Here's how the part is built. I have some questions about the finished solid (model axes, mm). A direction names the side the tool comes from. Coordinates: 2 decimals unless noted, no trailing zeros. Loops run counter-clockwise (first coordinate to the right, second up) from the corner with the lowest first, then second, coordinate; pieces in that order, holes last.
from build123d import *

# Parameters (mm, degrees)
SKETCH_1_W                  = 2300
SKETCH_1_H                  = 132
SM_BASE_FLANGE_1_DEPTH      = 1.6
SM_EDGE_FLANGE_1_DEPTH      = 2200
SM_EDGE_FLANGE_1_BEND_DEPTH = 2200
HOLE_WIZARD_6_4_6_4_1_D     = 6.4
HOLE_WIZARD_6_4_6_4_1_DEPTH = 2
CHAMFER_1_SIZE              = 50
CHAMFER_3_SIZE              = 10


# Sheet-metal steps are written as plain solids
with BuildPart() as part:
    # Sketch 1 → 基材-凸緣1 (new body)
    with BuildSketch(Plane(origin=(0, 0, 0), x_dir=(1, 0, 0), z_dir=(0, 1, 0))):
        Rectangle(SKETCH_1_W, SKETCH_1_H)
    extrude(amount=SM_BASE_FLANGE_1_DEPTH)

    # 邊線-凸緣1 section (across the edge) → 邊線-凸緣1 (add)
    with BuildSketch(Plane(origin=(1100, 1.6, -67), x_dir=(0, 0, 1), z_dir=(-1, 0, 0))):
        with BuildLine():
            Line((-1.6, 1), (-1.6, 60))
            Line((-1.6, 60), (0, 60))
            Line((0, 60), (0, 1))
            ThreePointArc((0, 1), (0.292893219, 0.292893219), (1, 0))
            Line((1, 0), (1, -1.6))
            ThreePointArc((1, -1.6), (-0.838477631, -0.838477631), (-1.6, 1))
        make_face()
    extrude(amount=SM_EDGE_FLANGE_1_DEPTH)

    # 邊線-凸緣1 section 2 (across the edge) → 邊線-凸緣1 bend (add)
    with BuildSketch(Plane(origin=(-1100, 1.6, 67), x_dir=(0, 0, -1), z_dir=(1, 0, 0))):
        with BuildLine():
            Line((-1.6, 1), (-1.6, 60))
            Line((-1.6, 60), (0, 60))
            Line((0, 60), (0, 1))
            ThreePointArc((0, 1), (0.292893219, 0.292893219), (1, 0))
            Line((1, 0), (1, -1.6))
            ThreePointArc((1, -1.6), (-0.838477631, -0.838477631), (-1.6, 1))
        make_face()
    extrude(amount=SM_EDGE_FLANGE_1_BEND_DEPTH)

    # Ø6.4 (6.4) 直徑孔1
    with Locations(Plane(origin=(0, 1.6, 0), x_dir=(-1, 0, 0), z_dir=(0, 1, 0))):
        with Locations((1110, -59), (1134, -59), (1134, 59), (1110, 59), (-1110, -59), (-1134, -59), (-1110, 59), (-1134, 59)):
            Hole(HOLE_WIZARD_6_4_6_4_1_D / 2, depth=HOLE_WIZARD_6_4_6_4_1_DEPTH)

    # 導角1
    chamfer_1_edges = [part.edges().sort_by_distance(p)[0] for p in [
        (1100, 61.6, -67.8),
        (-1100, 61.6, -67.8),
        (-1100, 61.6, 67.8),
        (1100, 61.6, 67.8),
    ]]
    chamfer(chamfer_1_edges, length=CHAMFER_1_SIZE)

    # 導角3
    chamfer_3_edges = [part.edges().sort_by_distance(p)[0] for p in [
        (-1150, 0.8, 66),
        (-1150, 0.8, -66),
        (1150, 0.8, -66),
        (1150, 0.8, 66),
    ]]
    chamfer(chamfer_3_edges, length=CHAMFER_3_SIZE)


solid = part.part
Q1. Will these pins go through, and if not, where does the flat tip stop? P1, Ø5, axis at x = 1134, z = 59, coming from the +Y side; P2, Ø6, axis at x = -249, z = 0, coming from the +Y side; P3, Ø1.8, axis at x = -1119, y = 1, coming from the +Z side; P4, Ø0.8, axis at y = 7, z = 67, coming from the +X side.
Q2. We'd pull the mould along Z, two halves only. Please class faces 1 (the flat face through (15, 33, -67)), 2 (the flat face through (-16, 1.6, -1)), 3 (the flat face through (-16, 0, -1)), 4 (the flat face through (-15, 32, 68.6)): pulls with the +Z half, pulls with the -Z half, needs draft (parallel to the pull), parting line crosses it, or undercut.
Q3. Suppose I cut it at A-A on y = 42.5. Write out the boundary of the cut face in (x, z), and give its area (3 significant figures).
Q4. Please list where these lines run through material, in increasing order: probe 1 along Z at (x, y) = (1110, 1.2); probe 2 along Z at (x, y) = (-913.5, 42); probe 3 along Y at (x, z) = (614.5, -18.5).
Q5. Suppose I cut it at B-B on x = 114. Write out the boundary of the cut face in (y, z).
Q6. For faces 5 (the flat face through (-15, 33, 67)), 6 (the flat face through (-1074.65, 36.95, -67.81)), which set-ups out of +Z, -Z, +X, -X, +Y, -Y let a thin tool reach every point of the face, with its end or its side?
Q7. Suppose I cut it at C-C on z = 9. Write out the boundary of the cut face in (x, y).
Check values:
1. P1: passes through
1. P2: stops at y = 1.6
1. P3: stops at z = 66
1. P4: stops at x = 1100
2. face 1: undercut
2. face 2: undercut
2. face 3: needs draft
2. face 4: pulls with the +Z half
3. outline: (-1069.1, -68.6) - (1069.1, -68.6) - (1069.1, -67) - (-1069.1, -67) - close; (-1069.1, 67) - (1069.1, 67) - (1069.1, 68.6) - (-1069.1, 68.6) - close
3. area: 6,840 mm2
4. probe 1: z = -66 to -62.2, -55.8 to 55.8, 62.2 to 66
4. probe 2: z = -68.6 to -67, 67 to 68.6
4. probe 3: y = 0 to 1.6
5. outline: (0, -66) arc R2.6 ccw to (2.6, -68.6) - (61.6, -68.6) - (61.6, -67) - (2.6, -67) arc R1 cw to (1.6, -66) - (1.6, 66) arc R1 cw to (2.6, 67) - (61.6, 67) - (61.6, 68.6) - (2.6, 68.6) arc R2.6 ccw to (0, 66) - close
6. face 5: +X, -X, +Y
6. face 6: +Z, -Z, -X, +Y
7. outline: (-1150, 0) - (1150, 0) - (1150, 1.6) - (-1150, 1.6) - close
